Here's how the part is built. I have some questions about the finished solid (model axes, mm). Give positions to 0.01 mm unless a question says otherwise; leave off trailing zeros. Write each loop counter-clockwise with the first axis right and the second up, starting at its lowest first coordinate (ties: lowest second). Pieces come first, ordered by that corner, then holes. Notation, with made-up numbers: (75, 88) - (107, 88) arc R7 ccw to (107, 93) - close; hole circle Ø8 at (35, 18.25). An arc over 180 degrees is marked (long way). Use a Markdown table: item, result.
Autodesk Inventor part; units mm, degrees
ref_plane "YZ Plane" through (0, 0, 0) normal (1, 0, 0) x (0, 1, 0)
ref_plane "XZ Plane" through (0, 0, 0) normal (0, 1, 0) x (-1, 0, 0)
ref_plane "XY Plane" through (0, 0, 0) normal (0, 0, 1) x (1, 0, 0)
sketch "Sketch1" plane through (0, 0, 0) normal (0, 0, 1) x (1, 0, 0)
  line L0 (0, 0) -> (-200, 0)
  line L1 (-200, 0) -> (-200, 50)
  line L2 (-200, 50) -> (0, 50)
  line L3 (0, 50) -> (0, 0)
  dimension "d0" = 200
  dimension "d1" = 50
extrude "Cuerpo" add sketch "Sketch1" along normal blind 2.1
sketch "Sketch2" plane through (0, 0, 0) normal (0, 0, -1) x (-1, 0, 0)
  line L0 (0, 0) -> (200, 0)
  line L1 (200, 0) -> (200, 50)
  line L2 (200, 50) -> (0, 50)
  line L3 (0, 50) -> (0, 0)
  line L4 (0, 0) -> (200, 0)
  line L5 (200, 0) -> (200, 50)
  line L6 (200, 50) -> (0, 50)
  line L7 (0, 50) -> (0, 0)
  line L8 (196.8, 3.2) -> (3.2, 3.2)
  line L9 (3.2, 3.2) -> (3.2, 46.8)
  line L10 (3.2, 46.8) -> (196.8, 46.8)
  line L11 (196.8, 46.8) -> (196.8, 3.2)
  dimension "d4" = 3.2
extrude "Ranura" add sketch "Sketch2" along normal blind 0.9 contours L8 L9 L10 L11
sketch "Sketch4" plane through (0, 0, 2.1) normal (0, 0, 1) x (1, 0, 0)
  line L0 (-200, 50) -> (0, 50)
  line L1 (-100, 50) -> (-100, 0)
  line L2 (-200, 0) -> (0, 0)
  point P0 (-100, 25)
hole "Rueda Externa" at (-100, 25, 2.1) direction (0, 0, -1) diameter 20.2 end through all
equation "\"d0\" = base_largo"
equation "\"d1\" = base_ancho"
equation "\"d2\" = tapa_grosor"
equation "\"d4\" = base_muros_grosor + general_margen"
equation "\"d5\" = tapa_ranura"
equation "\"d8\" = tapa_eje_diametro"
properties part number "Tapa"
Item 1: Thinking about a two-plate mould opening in X: for faces 1 (the flat face through (-101, 36, 2.1)), 2 (the cylindrical face through (-91.04, 20.34, 0.58)), which applies, +X half, -X half, draft (parallel to the pull), parting line (faces both ways), or undercut?
Values:
| item | result |
|---|---|
| face 1 | draft |
| face 2 | undercut |
Item 2: If we section it at B-B, the plane x = -100: Write out the boundary of the cut face in (y, z).
Values:
| item | result |
|---|---|
| outline | (0, 0) - (3.2, 0) - (3.2, -0.9) - (14.9, -0.9) - (14.9, 2.1) - (0, 2.1) - close; (35.1, -0.9) - (46.8, -0.9) - (46.8, 0) - (50, 0) - (50, 2.1) - (35.1, 2.1) - close |
Item 3: Will this pin go through, and if not, where does the flat tip stop? pin 1 Ø0.7 at (x, z) = (-141.5, -0.5) entering from +Y.
Values:
| item | result |
|---|---|
| pin 1 | stops at y = 46.8 |
Item 4: If we section it at A-A, the plane y = 25: Write out the boundary of the cut face in (x, z), plus the area to 3 significant figures.
Values:
| item | result |
|---|---|
| outline | (-200, 0) - (-196.8, 0) - (-196.8, -0.9) - (-110.1, -0.9) - (-110.1, 2.1) - (-200, 2.1) - close; (-89.9, -0.9) - (-3.2, -0.9) - (-3.2, 0) - (0, 0) - (0, 2.1) - (-89.9, 2.1) - close |
| area | 534 mm2 |
Item 5: If we section it at C-C, the plane z = 1.45: Write out the boundary of the cut face in (x, y), plus the area to 3 significant figures.
Values:
| item | result |
|---|---|
| outline | (-200, 0) - (0, 0) - (0, 50) - (-200, 50) - close; hole circle Ø20.2 at (-100, 25) |
| area | 9,680 mm2 |
Item 6: I need wall thicknesses on line 1 along X through (y, z) = (25, 1.2); line 2 along Y through (x, z) = (-100, 0.75); line 3 along X through (y, z) = (25, -0.1). Which ranges of each line are inside material? Lowest first, please. Write a range as [from, to].
Values:
| item | result |
|---|---|
| line 1 | x = [-200, -110.1], [-89.9, 0] |
| line 2 | y = [0, 14.9], [35.1, 50] |
| line 3 | x = [-196.8, -110.1], [-89.9, -3.2] |
